For this review, use the dimensioned drawing (mm, ordinates from the lowest corner) and the shaded views. A direction names the side the tool comes from. Round coordinates to 2 decimals unless told otherwise and drop trailing zeros. Write each loop counter-clockwise with the first axis right and the second up, starting at its lowest first coordinate (ties: lowest second). Pieces come first, ordered by that corner, then holes. Notation, with made-up numbers: M 5.25,61.5 L 39.25,61.5 A26 cw 39.25,95.5 Z; hole C 36,-10.75 d11. An arc over 180 degrees is marked long. Use one line per item in the form item = value. Start each with the question number.
Item 1: For P1, Ø12, axis at y = 61, z = 17, coming from the +X side; P2, Ø3, axis at y = 91.5, z = 22.5, coming from the +X side; P3, Ø1, axis at x = 81.5, z = 32.5, coming from the -Y side, all flat-tipped, find the tip position at first contact; note any pin that passes through.
Item 2: For the marked faces 1 and 2, list the 3-axis set-ups (+Z, -Z, +X, -X, +Y, -Y) from which the entire face can be reached by the end or side of a thin tool; tool diameter is ignored.
Item 3: Add section D-D (x = 125). State the section outline as (y, z) points.
Item 4: Draft analysis for pull direction Y (two halves, no side actions). For the marked faces 3 and 4, state which applies: released by +Y, released by -Y, zero draft, split by the parting line, or undercut.
Item 5: Add section C-C (z = 52.5). State the section outline as (x, y) points.
Item 6: Add section A-A (y = 99.06). State the section outline as (x, z) points, and give its area (3 significant figures).
Item 7: For line 1 (Z direction, x = 156, y = 44.5); line 2 (X direction, y = 99, z = 35), list the stretches that pass through material, from the lowest coordinate up. Write a range as [from, to].
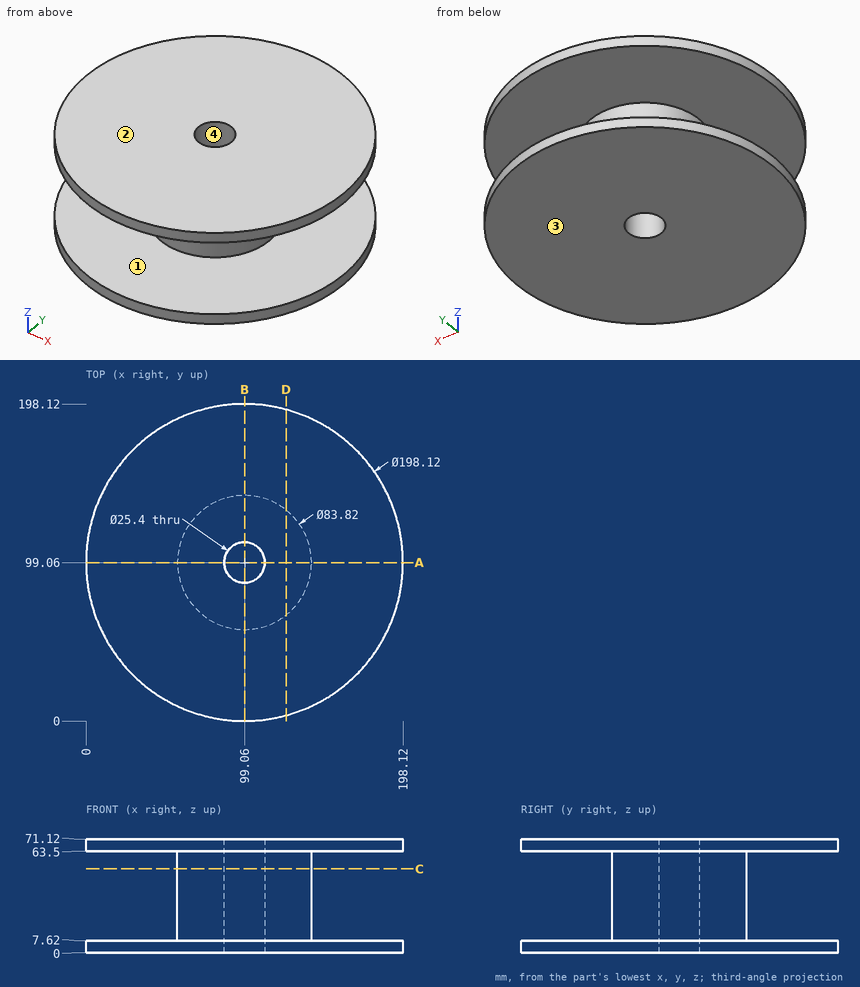
Calculated:
q1.P1 = 126.05
q1.P2 = 140.53
q1.P3 = 60.78
q2.face_1 = none
q2.face_2 = +Z, +X, -X, +Y, -Y
q3.outline = M 3.46,0 L 194.66,0 L 194.66,7.62 L 131.98,7.62 L 131.98,63.5 L 194.66,63.5 L 194.66,71.12 L 3.46,71.12 L 3.46,63.5 L 66.14,63.5 L 66.14,7.62 L 3.46,7.62 Z
q4.face_3 = zero draft
q4.face_4 = undercut
q5.outline = C 99.06,99.06 d83.82; hole C 99.06,99.06 d25.4
q6.outline = M 0,0 L 86.36,0 L 86.36,71.12 L 0,71.12 L 0,63.5 L 57.15,63.5 L 57.15,7.62 L 0,7.62 Z; M 111.76,0 L 198.12,0 L 198.12,7.62 L 140.97,7.62 L 140.97,63.5 L 198.12,63.5 L 198.12,71.12 L 111.76,71.12 Z
q6.area = 5,900 mm^2
q7.line_1 = [0, 7.62], [63.5, 71.12]
q7.line_2 = [57.15, 86.36], [111.76, 140.97]
